from build123d import *

# Parameters (mm, degrees)
F1_R     = 3.95
F2_DEPTH = 7
F3_R     = 6
F4_DEPTH = 1
F6_DEPTH = 2
F7_SIZE  = 0.5


with BuildPart() as f2:
    # F1 (on Top) → F2 (new body)
    with BuildSketch(Plane.XY):
        with Locations((-13.65, 0)):
            Circle(F1_R)
        with Locations((13.65, 0)):
            Circle(F1_R)
    extrude(amount=F2_DEPTH)

    # F3 (on face) → F4 (join)
    with BuildSketch(Plane(origin=(0, 0, 0), x_dir=(1, 0, 0), z_dir=(0, 0, -1))):
        with Locations((13.65, 0)):
            Circle(F3_R)
        with Locations((-13.65, 0)):
            Circle(F3_R)
    extrude(amount=F4_DEPTH)

    # F5 (on face) → F6 (join)
    with BuildSketch(Plane(origin=(0, 0, -1), x_dir=(1, 0, 0), z_dir=(0, 0, -1))):
        with BuildLine():
            ThreePointArc((-13.65, 11), (-24.65, 0), (-13.65, -11))
            Line((-13.65, -11), (13.65, -11))
            ThreePointArc((13.65, -11), (24.65, 0), (13.65, 11))
            Line((13.65, 11), (-13.65, 11))
        make_face()
    extrude(amount=F6_DEPTH)

    # F7
    f7_edges = [f2.edges().sort_by_distance(p)[0] for p in [
        (-17.6, 0, 7),
        (9.7, 0, 7),
    ]]
    chamfer(f7_edges, length=F7_SIZE)


solid = f2.part
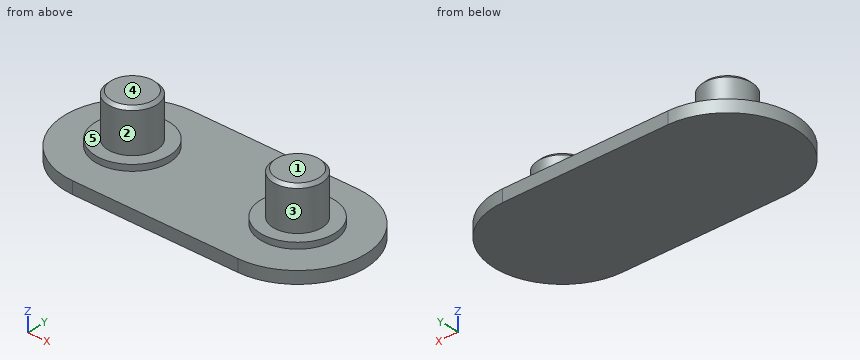
Design review of the part built by this model. Coordinates are the model's own, in mm. Face numbers are marked on the shaded views. A direction names the side the tool comes from. Give positions to 0.01 mm unless a question says otherwise; leave off trailing zeros. Write each loop counter-clockwise with the first axis right and the second up, starting at its lowest first coordinate (ties: lowest second). Pieces come first, ordered by that corner, then holes. Notation, with made-up numbers: M 89,22 L 119,22 A7 ccw 119,35 Z; hole C 7,85 d5. An arc over 180 degrees is marked long. Answer as a JSON object with one key per item and string values. Group by question number.
1) Tool access review of the marked faces 1 and 2: name each direction out of +Z, -Z, +X, -X, +Y, -Y from which nothing blocks a thin tool from reaching the whole face with its end or side.
2) We need section C-C (z = -2). Give the boundary of the cut face in (x, y).
3) Mouldability with a two-part tool opening along X and no side actions: class the marked faces 3, 4 and 5 as released by +X, released by -X, zero draft, split by the parting line, or undercut.
4) We need section B-B (x = 9). Give the boundary of the cut face in (y, z).
5) We need section D-D (y = -9). Give the boundary of the cut face in (x, z), and give its area (3 significant figures).
6) For line 1 along X through (y, z) = (0.25, 1); line 2 along Z through (x, y) = (9, 5.5); line 3 along Z through (x, y) = (-8.5, 1), list the stretches that pass through material, from the lowest coordinate up.
7) Clearance check with flat-ended pins moving along their axes: pin 1 Ø4 at (x, z) = (-10.5, 5) entering from +Y; pin 2 Ø6.5 at (x, y) = (-3, -0.5) entering from +Z; pin 3 Ø1.5 at (y, z) = (-5, 5.5) entering from -X; pin 4 Ø5 at (x, y) = (-7, 2) entering from +Z. State where each tip first meets the part, or that it passes through.
8) We need section A-A (z = 4.5). Give the boundary of the cut face in (x, y).
Answer key:
{
 "1": {"face 1": "+Z, +X, -X, +Y, -Y", "face 2": "+Z"},
 "2": {"outline": "M -13.65,-11 L 13.65,-11 A11 ccw 13.65,11 L -13.65,11 A11 ccw Z"},
 "3": {"face 3": "undercut", "face 4": "zero draft", "face 5": "undercut"},
 "4": {"outline": "M -11,-3 L 11,-3 L 11,-1 L 3.79,-1 L 3.79,0 L -3.79,0 L -3.79,-1 L -11,-1 Z"},
 "5": {"outline": "M -19.97,-3 L 19.97,-3 L 19.97,-1 L -19.97,-1 Z", "area": "79.9 mm²"},
 "6": {"line 1": "x = -17.59 to -9.71, 9.71 to 17.59", "line 2": "z = -3 to -1", "line 3": "z = -3 to 0"},
 "7": {"pin 1": "stops at y = 3.78", "pin 2": "stops at z = -1", "pin 3": "passes through", "pin 4": "stops at z = 0"},
 "8": {"outline": "C -13.65,0 d7.9; C 13.65,0 d7.9"}
}
